For this review, take the finished solid that the model builds, in its own axes (mm). Face numbers are marked on the shaded views. A direction names the side the tool comes from. Give positions to 0.01 mm unless a question says otherwise; leave off trailing zeros. Loops run counter-clockwise (first coordinate to the right, second up) from the corner with the lowest first, then second, coordinate; pieces in that order, holes last. Notation, with made-up numbers: M 12,51.5 L 25,51.5 A30 ccw 25,77.5 Z; hole C 88.25,83 d7. An arc over 180 degrees is marked long. Use CSV: the item, a comma, the result in double quotes. Start each with the question number.
1. The part is to be moulded in two halves that separate along X. For the marked faces 3, 4, 5 and 6, say which applies: pulls with the +X half, pulls with the -X half, needs draft (parallel to the pull), parting line crosses it, or undercut.
2. Take a section at B-B, the plane x = 0. Write out the cut boundary in (y, z).
3. Take a section at A-A, the plane z = 0. Write out the cut boundary in (x, y), and give its area (3 significant figures).
4. Take a section at C-C, the plane y = 4.5. Write out the cut boundary in (x, z), and give its area (3 significant figures).
5. Insertion check: P1, Ø4, axis at x = 0.5, z = -12, coming from the -Y side; P2, Ø5, axis at y = 1.5, z = 8.5, coming from the -X side; P3, Ø5, axis at y = 8, z = -10, coming from the -X side; P4, Ø2, axis at x = -16, y = 3, coming from the +Z side. Each pin has a flat end and moves straight along its axis. Give the tip position at first contact, or say it passes through.
6. To check wall thickness, follow line 1 (Z direction, x = 0, y = 4.5); line 2 (Z direction, x = 2.5, y = 4); line 3 (X direction, y = 7.25, z = 3.5). State the ranges of each line that lie inside material, in increasing order. Write a range as [from, to].
7. Take a section at D-D, the plane z = -12. Write out the cut boundary in (x, y), and give its area (3 significant figures).
8. Tool access review of the marked faces 1 and 2: name each direction out of +Z, -Z, +X, -X, +Y, -Y from which nothing blocks a thin tool from reaching the whole face with its end or side.
Autodesk Inventor part; units mm, degrees
ref_plane "YZ Plane" through (0, 0, 0) normal (1, 0, 0) x (0, 1, 0)
ref_plane "XZ Plane" through (0, 0, 0) normal (0, 1, 0) x (-1, 0, 0)
ref_plane "XY Plane" through (0, 0, 0) normal (0, 0, 1) x (1, 0, 0)
sketch "Sketch1" plane through (0, 0, 0) normal (0, 1, 0) x (-1, 0, 0)
  circle A0 centre (0, 0) radius 4.7674
  circle A1 centre (0, 0) radius 15
  line L0 (14.8106, 2.3764) -> (14.8106, -2.3764)
  line L1 (14.8106, -2.3764) -> (17.5065, -2.3764)
  line L2 (17.5065, -2.3764) -> (17.5065, 2.3764)
  line L3 (17.5065, 2.3764) -> (14.8106, 2.3764)
  dimension "d0" = 30
  dimension "d1" = 9.5349
extrude "Extrusion1" add sketch "Sketch1" along normal blind 10
properties part number "Test_gear_p2"
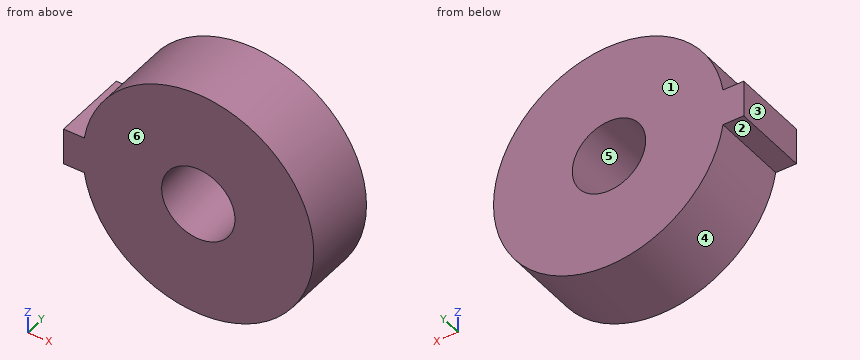
Result set:
1,face 3,"pulls with the -X half"
1,face 4,"parting line crosses it"
1,face 5,"undercut"
1,face 6,"needs draft"
2,outline,"M 0,-15 L 10,-15 L 10,-4.77 L 0,-4.77 Z; M 0,4.77 L 10,4.77 L 10,15 L 0,15 Z"
3,outline,"M -17.51,0 L -4.77,0 L -4.77,10 L -17.51,10 Z; M 4.77,0 L 15,0 L 15,10 L 4.77,10 Z"
3,area,"230 mm2"
4,outline,"M -17.51,-2.38 L -14.81,-2.38 A15 ccw long -14.81,2.38 L -17.51,2.38 Z; hole C 0,0 d9.53"
4,area,"648 mm2"
5,P1,"y = 0"
5,P2,"x = -13.75"
5,P3,"x = -12.99"
5,P4,"z = 2.38"
6,line 1,"[-15, -4.77], [4.77, 15]"
6,line 2,"[-14.79, -4.06], [4.06, 14.79]"
6,line 3,"[-14.59, -3.24], [3.24, 14.59]"
7,outline,"M -9,0 L 9,0 L 9,10 L -9,10 Z"
7,area,"180 mm2"
8,face 1,"+Z, -Z, +X, -X, +Y"
8,face 2,"-Z, -X, +Y, -Y"
